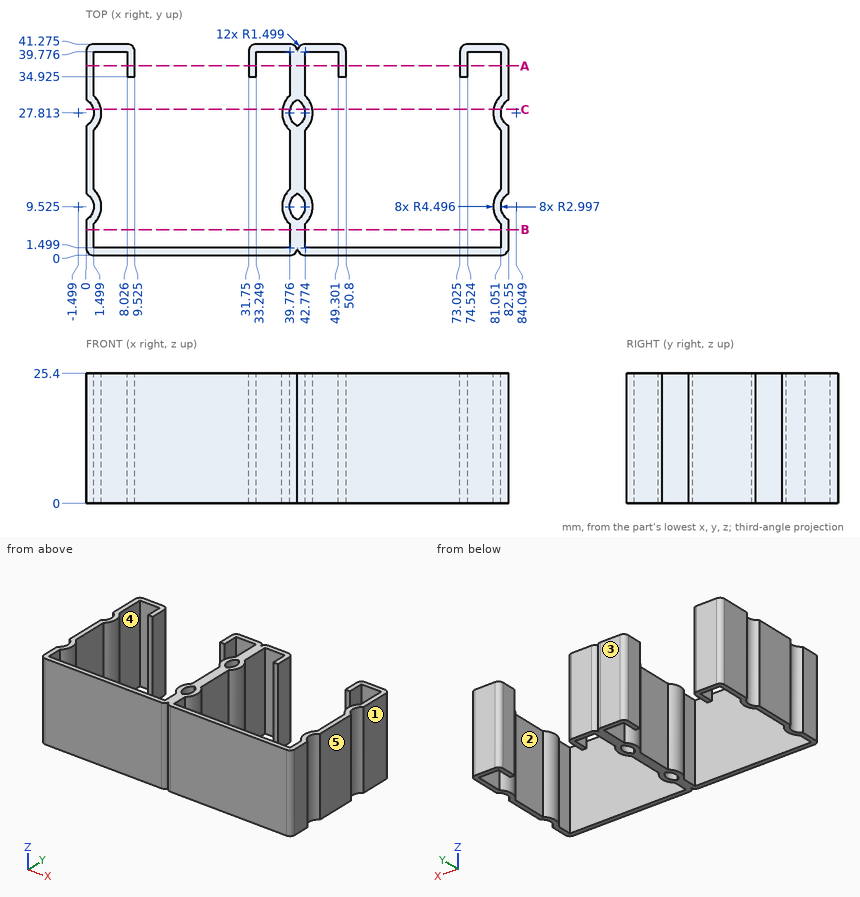
Job drawing, mm, ordinate dimensions from the low corner. One solid piece. A direction names the side the tool comes from. Coordinates: 2 decimals unless noted, no trailing zeros. Order: outer loops, then holes, each group sorted by start corner. A loop starts at its lowest first (then second) coordinate and runs counter-clockwise, first axis right, second up. Notation, with made-up numbers: (-34, 55) - (-16, 55) arc R14 ccw to (-16, 81) - close; hole circle Ø5 at (-5.5, 14). An arc over 180 degrees is marked (long way). Write each question's results on one line, items separated by ' | '. Start each with the question number.
Item 1: Mould opens along Y. For the marked faces 3, 4 and 5 say: released by +Y, released by -Y, zero draft, split by the parting line, or undercut.
Item 2: Tool access for the marked faces 1 and 2: list every direction of +Z, -Z, +X, -X, +Y, -Y with a clear straight run to the whole face (end or side of a thin tool).
Item 3: Band-saw the part on B-B on y = 5. Write the cut outline in (x, z).
Item 4: Flat gauge pins, fed straight in: pin 1 (6 mm diameter, centred on x = 15.5, z = 7, fed in from +Y); pin 2 (6 mm diameter, centred on x = 31, y = 31, fed in from +Z). Where does each tip first touch, or does it go through?
Item 5: Wall check: probe 1 along X at (y, z) = (5.5, 24); probe 2 along Y at (x, z) = (37, 12) (1 decimal); probe 3 along X at (y, z) = (10.5, 7) (1 decimal). Give the ranges that are in metal, low to high. Write a range as [from, to].
Item 6: Band-saw the part on A-A on y = 37. State how many separate pieces and enclosed holes the cut face has.
Item 7: Band-saw the part on C-C on y = 28.5. Write the cut outline in (x, z) (1 decimal), and give its area (3 significant figures).
Numbers:
1) face 3: released by +Y | face 4: undercut | face 5: zero draft
2) face 1: +Z, -Z, +X, +Y, -Y | face 2: +Z, -Z
3) outline: (0, 0) - (1.5, 0) - (1.5, 25.4) - (0, 25.4) - close; (39.78, 0) - (42.77, 0) - (42.77, 25.4) - (39.78, 25.4) - close; (81.05, 0) - (82.55, 0) - (82.55, 25.4) - (81.05, 25.4) - close
4) pin 1: y = 1.5 | pin 2: through
5) probe 1: [0, 1.5], [39.78, 42.77], [81.05, 82.55] | probe 2: [0, 1.5], [39.8, 41.3] | probe 3: [1.3, 2.9], [38.4, 39.9], [42.6, 44.2], [79.7, 81.2]
6) separate pieces: 7 | enclosed holes: 0
7) outline: (1.4, 0) - (2.9, 0) - (2.9, 25.4) - (1.4, 25.4) - close; (38.3, 0) - (39.9, 0) - (39.9, 25.4) - (38.3, 25.4) - close; (42.7, 0) - (44.2, 0) - (44.2, 25.4) - (42.7, 25.4) - close; (79.6, 0) - (81.1, 0) - (81.1, 25.4) - (79.6, 25.4) - close | area: 155 mm^2
